from build123d import *

# Parameters (mm, degrees)
SKETCH1_R           = 15
BOSS_EXTRUDE1_DEPTH = 10
BOSS_EXTRUDE1_DRAFT = -5
SKETCH3_R           = 5
CUT_EXTRUDE1_DEPTH  = 5
FILLET1_R           = 2


with BuildPart() as part:
    # Sketch1 → Boss-Extrude1 (with draft: the straight prism first)
    with BuildSketch(Plane(origin=(0, 0, 0), x_dir=(1, 0, 0), z_dir=(0, 1, 0))):
        Circle(SKETCH1_R)
    extrude(amount=-BOSS_EXTRUDE1_DEPTH)
    # Boss-Extrude1: the draft: its side faces are tilted about the plane it starts from
    boss_extrude1_sides = [part.faces().sort_by_distance(p)[0] for p in [
        (-15, -5, 0),
    ]]
    draft(boss_extrude1_sides, Plane(origin=(0, 0, 0), x_dir=(1, 0, 0), z_dir=(0, 1, 0)), BOSS_EXTRUDE1_DRAFT)

    # Boss-Extrude2 cone 1 section (through the dimple's axis) → Boss-Extrude2 (revolve)
    with BuildSketch(Plane(origin=(0, 0, -7.5), x_dir=(0, 0, -1), z_dir=(1, 0, 0))):
        Polygon((0, 0), (2.5, 0), (0, 14.178204549), align=None)
    revolve(axis=Axis((0, 0, -7.5), (0, 1, 0)))

    # Boss-Extrude2 cone 2 section (through the dimple's axis) → Boss-Extrude2 cone 2 (revolve)
    with BuildSketch(Plane(origin=(7.5, 0, 0), x_dir=(0, 0, -1), z_dir=(1, 0, 0))):
        Polygon((0, 0), (2.5, 0), (0, 14.178204549), align=None)
    revolve(axis=Axis((7.5, 0, 0), (0, 1, 0)))

    # Boss-Extrude2 cone 3 section (through the dimple's axis) → Boss-Extrude2 cone 3 (revolve)
    with BuildSketch(Plane(origin=(0, 0, 7.5), x_dir=(0, 0, -1), z_dir=(1, 0, 0))):
        Polygon((0, 0), (2.5, 0), (0, 14.178204549), align=None)
    revolve(axis=Axis((0, 0, 7.5), (0, 1, 0)))

    # Boss-Extrude2 cone 4 section (through the dimple's axis) → Boss-Extrude2 cone 4 (revolve)
    with BuildSketch(Plane(origin=(-7.5, 0, 0), x_dir=(0, 0, -1), z_dir=(1, 0, 0))):
        Polygon((0, 0), (2.5, 0), (0, 14.178204549), align=None)
    revolve(axis=Axis((-7.5, 0, 0), (0, 1, 0)))

    # Sketch3 → Cut-Extrude1 (cut)
    with BuildSketch(Plane(origin=(0, -10, 0), x_dir=(-1, 0, 0), z_dir=(0, -1, 0))):
        with Locations(Location((0, 0, 0), (0, 0, 90))):
            Circle(SKETCH3_R)
    extrude(amount=-CUT_EXTRUDE1_DEPTH, mode=Mode.SUBTRACT)

    # Fillet1
    fillet1_edges = [part.edges().sort_by_distance(p)[0] for p in [
        (-15, 0, 0),
        (-14.125113365, -10, 0),
    ]]
    fillet(fillet1_edges, radius=FILLET1_R)


solid = part.part
Verification items for the finished model (mm, model axes). A direction names the side the tool comes from. Give positions to 0.01 mm unless a question says otherwise; leave off trailing zeros. Write each loop counter-clockwise with the first axis right and the second up, starting at its lowest first coordinate (ties: lowest second). Pieces come first, ordered by that corner, then holes. Notation, with made-up numbers: M -6.5,31 L 17.5,31 A7 cw 17.5,43 Z; hole C -9,12 d10. An arc over 180 degrees is marked long. Write item = value, one per line.
(1) Sectioned sample at B-B (y = -6.75). Record the cut outline in (x, z), then the cut area to 3 significant figures.
Found:
outline = C 0,0 d28.82; hole C 0,0 d10
area = 574 mm2
(2) Access from +Z, -Z, +X, -X, +Y, -Y to the whole of each face (thin tool, end or side, straight path). Record for faces 4 (the face through (0, -5, 0)), 5 (the face through (0, 0, 0)).
Found:
face_4 = -Y
face_5 = +Y
(3) Sectioned sample at A-A (y = 3.5). Record the cut outline in (x, z), then the cut area to 3 significant figures.
Found:
outline = C -7.5,0 d3.77; C 0,-7.5 d3.77; C 0,7.5 d3.77; C 7.5,0 d3.77
area = 44.5 mm2
(4) Draft check along Z on faces 1 (the face through (-8.72, 7.19, 0.16)), 2 (the face through (-4.88, -7.54, 1.08)), 3 (the face through (-0.2, -10, 5.3)). Enter one of: released by +Z, released by -Z, zero draft, split by the parting line, or undercut.
Found:
face_1 = split by the parting line
face_2 = undercut
face_3 = zero draft
(5) Go/stop test with flat-tipped pins: pin 1 Ø1.5 at (y, z) = (-6.5, -5.5) entering from -X; pin 2 Ø2 at (x, y) = (4.5, -5.5) entering from +Z; pin 3 Ø9 at (x, z) = (0, 0) entering from +Y. Record where each tip stops, or that it passes through.
Found:
pin_1 = -13.64
pin_2 = 14.11
pin_3 = 0
(6) Material ranges on line 1 (Y direction, x = 2.5, z = -0.5); line 2 (Y direction, x = -2.75, z = -11); line 3 (X direction, y = -7.25, z = 0), recorded low to high.
Found:
line_1 = -5 to 0
line_2 = -10 to 0
line_3 = -14.37 to -5, 5 to 14.37
(7) Sectioned sample at C-C (y = 0.75). Record the cut outline in (x, z), then the cut area to 3 significant figures.
Found:
outline = C -7.5,0 d4.74; C 0,-7.5 d4.74; C 0,7.5 d4.74; C 7.5,0 d4.74
area = 70.5 mm2
